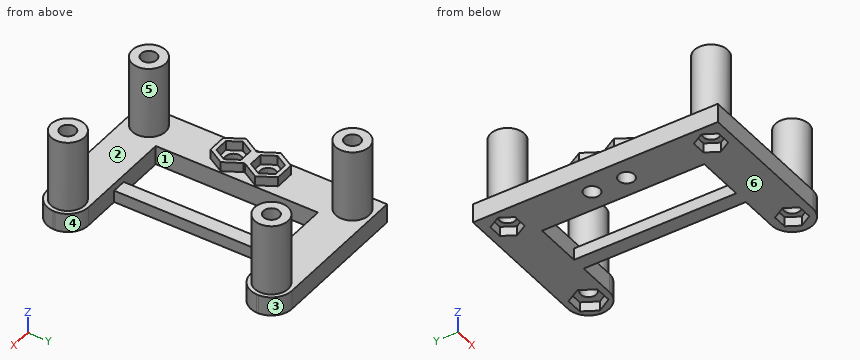
Autodesk Inventor part; units mm, degrees
ref_plane "YZ Plane" through (0, 0, 0) normal (1, 0, 0) x (0, 1, 0)
ref_plane "XZ Plane" through (0, 0, 0) normal (0, 1, 0) x (-1, 0, 0)
ref_plane "XY Plane" through (0, 0, 0) normal (0, 0, 1) x (1, 0, 0)
sketch "Sketch1" plane through (0, 0, 0) normal (0, 0, 1) x (1, 0, 0)
  line L0 (0, 0) -> (41.5, 0)
  line L1 (41.5, 0) -> (41.5, -73)
  line L2 (41.5, -73) -> (0, -73)
  line L3 (0, -73) -> (0, 0)
  line L4 (0, -73) -> (3.11, -73)
  line L5 (0, -73) -> (3.11, -73) construction
  line L6 (3.11, -73) -> (3.11, -69.85)
  line L7 (3.11, -73) -> (6.26, -73) construction
  line L8 (3.11, -69.85) -> (14.54, -69.85)
  line L9 (14.54, -69.85) -> (19.65, -69.85)
  line L10 (19.65, -69.85) -> (31.08, -69.85)
  circle A0 centre (3.11, -69.85) radius 1.6
  circle A1 centre (14.54, -69.85) radius 1.6
  circle A2 centre (19.65, -69.85) radius 1.6
  circle A3 centre (31.08, -69.85) radius 1.6
  line L11 (3.11, -69.85) -> (3.11, -55.42)
  line L12 (3.11, -69.85) -> (17.54, -69.85) construction
  line L13 (0, -73) -> (4.33, -73)
  line L14 (0, -73) -> (4.33, -73) construction
  line L15 (4.33, -73) -> (4.33, -53.49)
  line L16 (3.11, -55.42) -> (6.6479, -55.42)
  circle A4 centre (4.33, -55.42) radius 1.651
  line L17 (4.33, -55.42) -> (4.33, -37.69)
  line L18 (4.33, -55.42) -> (22.06, -55.42) construction
  line L19 (4.33, -55.42) -> (29.68, -55.42)
  line L20 (4.33, -55.42) -> (29.68, -55.42) construction
  circle A5 centre (4.33, -37.69) radius 1.651
  circle A6 centre (29.68, -55.42) radius 1.651
  line L21 (4.33, -37.69) -> (39.0376, -37.69)
  line L22 (29.68, -55.42) -> (29.68, -25.3245)
  circle A7 centre (29.68, -37.69) radius 1.651
  line L23 (4.33, -37.69) -> (4.33, -30.44)
  line L24 (4.33, -37.69) -> (11.58, -37.69) construction
  line L25 (4.33, -30.44) -> (4.33, -12.71)
  line L26 (4.33, -30.44) -> (29.68, -30.44)
  line L27 (4.33, -30.44) -> (29.68, -30.44) construction
  line L28 (4.33, -12.71) -> (29.68, -12.71)
  circle A8 centre (29.68, -12.71) radius 1.651
  circle A9 centre (4.33, -12.71) radius 1.651
  circle A10 centre (4.33, -30.44) radius 1.651
  circle A11 centre (29.68, -30.44) radius 1.651
  line L29 (29.68, -12.71) -> (29.68, -11.3536)
  dimension "d0" = 41.5
  dimension "d1" = 73
  dimension "d2" = 3.11
  dimension "d3" = 0
  dimension "d4" = 3.15
  dimension "d5" = 90
  dimension "d6" = 11.43
  dimension "d7" = 90
  dimension "d9" = 5.11
  dimension "d10" = 11.43
  dimension "d11" = 180
  dimension "d12" = 3.2
  dimension "d13" = 3.2
  dimension "d14" = 3.2
  dimension "d15" = 3.2
  dimension "d18" = 14.43
  dimension "d19" = 90
  dimension "d20" = 4.33
  dimension "d21" = 0
  dimension "d22" = 3.302
  dimension "d23" = 17.73
  dimension "d24" = 90
  dimension "d25" = 25.35
  dimension "d26" = 0
  dimension "d27" = 3.302
  dimension "d28" = 3.302
  dimension "d29" = 3.302
  dimension "d30" = 7.25
  dimension "d31" = 90
  dimension "d32" = 17.73
  dimension "d33" = 180
  dimension "d34" = 25.35
  dimension "d35" = 0
  dimension "d36" = 25.35
  dimension "d37" = 3.302
  dimension "d38" = 3.302
  dimension "d39" = 3.302
  dimension "d40" = 3.302
extrude "Extrusion2" add sketch "Sketch1" along normal blind 4 contours L0 L1 L2 L15 A0 A4 L16 L19 A6 L22 A7 A11 L26 A10 L23 A5 L17 L11 L6 L3 | L6 A0 L15 L2 | L11 A4 L15 A0 | L15 L17 A5 L21 A7 L22 A6 L19 L16 A4 | L23 A10 L26 A11 L22 A7 L21 A5
sketch "Sketch3" plane through (0, 0, 4) normal (0, 0, 1) x (1, 0, 0)
  circle A0 centre (4.33, -55.42) radius 1.651
  circle A1 centre (4.33, -55.42) radius 3.5
  circle A2 centre (29.68, -55.42) radius 1.651
  circle A3 centre (29.68, -55.42) radius 3.5
  circle A4 centre (4.33, -12.71) radius 1.651
  circle A5 centre (4.33, -12.71) radius 3.5
  circle A6 centre (29.68, -12.71) radius 1.651
  circle A7 centre (29.68, -12.71) radius 3.5
  point P0 (0, 0)
  dimension "d46" = 7
  dimension "d47" = 7
  dimension "d48" = 7
  dimension "d49" = 7
extrude "Extrusion4" add sketch "Sketch3" along normal blind 15
sketch "Sketch8" plane through (0, 0, 0) normal (0, 0, -1) x (-1, 0, 0)
  circle A0 centre (-4.33, -12.71) radius 1.651
  circle A1 centre (-4.33, -12.71) radius 3
  circle A2 centre (-29.68, -12.71) radius 1.651
  circle A3 centre (-29.68, -12.71) radius 3
  circle A4 centre (-29.68, -55.42) radius 1.651
  circle A5 centre (-29.68, -55.42) radius 3
  circle A6 centre (-4.33, -55.42) radius 1.651
  circle A7 centre (-4.33, -55.42) radius 3
  line L0 (-1.33, -12.71) -> (-2.83, -15.3081)
  line L1 (-2.83, -15.3081) -> (-5.83, -15.3081)
  line L2 (-5.83, -15.3081) -> (-7.33, -12.71)
  line L3 (-7.33, -12.71) -> (-5.83, -10.1119)
  line L4 (-5.83, -10.1119) -> (-2.83, -10.1119)
  line L5 (-2.83, -10.1119) -> (-1.33, -12.71)
  circle A8 centre (-29.68, -12.71) radius 3.5
  line L6 (-26.18, -12.6978) -> (-27.9194, -15.735)
  line L7 (-27.9194, -15.735) -> (-31.4194, -15.7472)
  line L8 (-31.4194, -15.7472) -> (-33.18, -12.7222)
  line L9 (-33.18, -12.7222) -> (-31.4406, -9.685)
  line L10 (-31.4406, -9.685) -> (-27.9406, -9.6728)
  line L11 (-27.9406, -9.6728) -> (-26.18, -12.6978)
  line L12 (-26.68, -55.42) -> (-28.18, -58.0181)
  line L13 (-28.18, -58.0181) -> (-31.18, -58.0181)
  line L14 (-31.18, -58.0181) -> (-32.68, -55.42)
  line L15 (-32.68, -55.42) -> (-31.18, -52.8219)
  line L16 (-31.18, -52.8219) -> (-28.18, -52.8219)
  line L17 (-28.18, -52.8219) -> (-26.68, -55.42)
  line L18 (-1.3301, -55.3946) -> (-2.808, -58.0053)
  line L19 (-2.808, -58.0053) -> (-5.8079, -58.0307)
  line L20 (-5.8079, -58.0307) -> (-7.3299, -55.4454)
  line L21 (-7.3299, -55.4454) -> (-5.852, -52.8347)
  line L22 (-5.852, -52.8347) -> (-2.8521, -52.8093)
  line L23 (-2.8521, -52.8093) -> (-1.3301, -55.3946)
  point P0 (0, 0)
  dimension "d53" = 6
  dimension "d55" = 6
  dimension "d56" = 6
  dimension "d54" = 6
extrude "Extrusion5" cut sketch "Sketch8" against normal blind 2 contours L0 L1 L2 L3 L4 L5 | A2 | A3 | L12 L13 L14 L15 L16 L17 | L18 L19 L20 L21 L22 L23 | L6 L7 L8 L9 L10 L11
sketch "Sketch9" plane through (0, 0, 4) normal (0, 0, 1) x (1, 0, 0)
  circle A0 centre (4.33, -30.44) radius 1.651
  circle A1 centre (4.33, -30.44) radius 1.651
  circle A2 centre (4.33, -37.69) radius 1.651
  circle A3 centre (4.33, -37.69) radius 1.651
  line L0 (7.33, -30.44) -> (5.83, -33.0381)
  line L1 (5.83, -33.0381) -> (2.83, -33.0381)
  line L2 (2.83, -33.0381) -> (1.33, -30.44)
  line L3 (1.33, -30.44) -> (2.83, -27.8419)
  line L4 (2.83, -27.8419) -> (5.83, -27.8419)
  line L5 (5.83, -27.8419) -> (7.33, -30.44)
  line L6 (7.33, -37.69) -> (5.83, -40.2881)
  line L7 (5.83, -40.2881) -> (2.83, -40.2881)
  line L8 (2.83, -40.2881) -> (1.33, -37.69)
  line L9 (1.33, -37.69) -> (2.83, -35.0919)
  line L10 (2.83, -35.0919) -> (5.83, -35.0919)
  line L11 (5.83, -35.0919) -> (7.33, -37.69)
  line L12 (8.33, -30.44) -> (6.33, -33.9041)
  line L13 (6.33, -33.9041) -> (2.33, -33.9041)
  line L14 (2.33, -33.9041) -> (0.33, -30.44)
  line L15 (0.33, -30.44) -> (2.33, -26.9759)
  line L16 (2.33, -26.9759) -> (6.33, -26.9759)
  line L17 (6.33, -26.9759) -> (8.33, -30.44)
  line L18 (8.33, -37.69) -> (6.33, -41.1541)
  line L19 (6.33, -41.1541) -> (2.33, -41.1541)
  line L20 (2.33, -41.1541) -> (0.33, -37.69)
  line L21 (0.33, -37.69) -> (2.33, -34.2259)
  line L22 (2.33, -34.2259) -> (6.33, -34.2259)
  line L23 (6.33, -34.2259) -> (8.33, -37.69)
  line L24 (6.33, -33.9041) -> (6.33, -34.2259)
  line L25 (2.33, -33.9041) -> (2.33, -34.2259)
  point P0 (0, 0)
  dimension "d59" = 3.302
  dimension "d60" = 3.302
extrude "Extrusion6" add sketch "Sketch9" along normal blind 2 contours L12 L13 L14 L15 L16 L17 | L24 L22 L25 L13 | L23 L18 L19 L20 L21 L22
sketch "Sketch10" plane through (0, 0, 0) normal (0, 0, -1) x (-1, 0, 0)
  circle A0 centre (-4.33, -55.42) radius 1.651
  circle A1 centre (-4.33, -12.71) radius 3.5
  circle A2 centre (-4.33, -12.71) radius 4.33
  line L0 (-4.33, -8.38) -> (6.0992, -8.38)
  line L1 (-4.33, -8.38) -> (-46.273, -8.38)
  circle A3 centre (-29.68, -55.42) radius 1.651
  circle A4 centre (-29.68, -12.71) radius 1.651
  circle A5 centre (-29.68, -12.71) radius 4.33
  line L2 (-34.01, -12.71) -> (-34.01, 23.2585)
  circle A6 centre (-4.33, -55.42) radius 4.33
  line L3 (-34.01, -12.71) -> (-34.01, -66.3278)
  line L4 (-4.33, -59.75) -> (-38.3543, -59.75)
  circle A7 centre (-29.68, -55.42) radius 4.33
  line L5 (-29.68, -55.42) -> (-29.68, -12.71)
  circle A8 centre (-4.33, -12.71) radius 1.651
  line L6 (-4.33, -12.71) -> (-29.68, -12.71)
  line L7 (-18.2288, -59.75) -> (-46.273, -59.75)
  line L8 (-46.273, -59.75) -> (-46.273, -78.0952)
  line L9 (-46.273, -78.0952) -> (-18.2288, -78.0952)
  line L10 (-18.2288, -78.0952) -> (-18.2288, -59.75)
  line L11 (-18.2288, -59.75) -> (2.2846, -59.75)
  line L12 (2.2846, -59.75) -> (2.2846, -79.2844)
  line L13 (2.2846, -79.2844) -> (-18.2288, -79.2844)
  line L14 (-18.2288, -79.2844) -> (-18.2288, -59.75)
  line L15 (-34.01, -59.75) -> (-49.3705, -59.75)
  line L16 (-49.3705, -59.75) -> (-49.3705, 18.5259)
  line L17 (-49.3705, 18.5259) -> (-34.01, 18.5259)
  line L18 (-34.01, 18.5259) -> (-34.01, -59.75)
  line L19 (-34.01, -8.38) -> (8.0076, -8.38)
  line L20 (8.0076, -8.38) -> (8.0076, 15.8503)
  line L21 (8.0076, 15.8503) -> (-34.01, 15.8503)
  line L22 (-34.01, 15.8503) -> (-34.01, -8.38)
  point P0 (0, 0)
extrude "Extrusion7" cut sketch "Sketch10" along normal mid plane 100 contours L1 L2 L21 L20 L19 L0 | L2 L3 L4 L7 L15 L16 L17 | L4 L10 L9 L8 L7 | L4 L11 L12 L13 L14 L10
sketch "Sketch11" plane through (0, 0, 0) normal (0, 0, -1) x (-1, 0, 0)
  line L0 (-34.01, -59.75) -> (0, -59.75)
  line L1 (0, -8.38) -> (-34.01, -8.38)
  circle A0 centre (-4.33, -55.42) radius 1.651
  circle A1 centre (-4.33, -55.42) radius 4.3403
  circle A2 centre (-4.33, -12.71) radius 1.651
  circle A3 centre (-4.33, -12.71) radius 4.3403
  line L2 (-4.3352, -51.0797) -> (-29.68, -51.0797)
  line L3 (-29.68, -59.75) -> (-4.3352, -59.75)
  line L4 (-4.3352, -59.75) -> (-4.3352, -51.0797)
  line L5 (-4.3352, -17.0503) -> (-29.68, -17.0503)
  line L6 (-29.68, -8.38) -> (-4.3352, -8.38)
  line L7 (-4.3352, -8.38) -> (-4.3352, -17.0503)
  line L8 (-4.3352, -51.0797) -> (-8.6703, -51.0797)
  line L9 (-8.6703, -51.0797) -> (-8.6703, -12.7152)
  line L10 (-8.6703, -12.7152) -> (-4.3352, -12.7152)
  line L11 (-4.3352, -12.7152) -> (-4.3352, -51.0797)
  line L12 (-34.01, -8.38) -> (-34.01, -59.75)
  line L13 (-8.6703, -17.0503) -> (-34.01, -17.0503)
  line L14 (-34.01, -17.0503) -> (-34.01, -51.0797)
  line L15 (-34.01, -51.0797) -> (-8.6703, -51.0797)
  line L16 (-8.6703, -51.0797) -> (-8.6703, -17.0503)
  line L17 (-29.68, -59.75) -> (-36.7019, -59.75)
  line L18 (-36.7019, -59.75) -> (-36.7019, -51.0797)
  line L19 (-36.7019, -51.0797) -> (-29.68, -51.0797)
  line L20 (-29.68, -17.0503) -> (-34.01, -17.0503)
  line L21 (-34.01, -17.0503) -> (-34.01, -8.38)
  line L22 (-34.01, -8.38) -> (-29.68, -8.38)
  arc A4 (-29.68, -51.0797) -> (-29.68, -59.75) centre (-29.68, -55.4148) ccw
  arc A5 (-29.68, -8.38) -> (-29.68, -17.0503) centre (-29.68, -12.7152) ccw
  line L23 (-29.68, -17.0503) -> (-40.5173, -17.0503)
  line L24 (-40.5173, -17.0503) -> (-40.5173, -8.38)
  line L25 (-40.5173, -8.38) -> (-29.68, -8.38)
  line L26 (-8.6703, -51.0797) -> (-41.5169, -51.0797)
  line L27 (-41.5169, -51.0797) -> (-41.5169, -17.0503)
  line L28 (-41.5169, -17.0503) -> (-8.6703, -17.0503)
  line L29 (-8.6703, -17.0503) -> (-8.6703, -51.0797)
  arc A6 (-29.68, -8.38) -> (-29.68, -17.0503) centre (-29.68, -12.7152) ccw
  line L30 (-29.68, -8.38) -> (-34.01, -8.38)
  point P0 (0, 0)
  point P1 (-29.68, -55.42)
extrude "Extrusion8" cut sketch "Sketch11" along normal mid plane 100 contours L12 A4 L0 | L17 L18 L19 L12 A4 | L12 L15 A4 | L12 L13 L5 L9 L2 L15 | L23 L24 L25 L12 A5 | L12 A5 L13 | L12 L1 A5
sketch "Sketch12" plane through (0, 0, 0) normal (0, 0, -1) x (-1, 0, 0)
  line L0 (-29.68, -51.0797) -> (-8.6703, -51.0797)
  line L1 (-8.6703, -17.0503) -> (-29.68, -17.0503)
  line L2 (-8.6703, -51.0797) -> (-18.6703, -51.0797)
  line L3 (-18.6703, -51.0797) -> (-18.6703, -17.0503)
  line L4 (-18.6703, -17.0503) -> (-8.6703, -17.0503)
  line L5 (-8.6703, -17.0503) -> (-8.6703, -51.0797)
  line L6 (-18.6703, -17.0503) -> (-21.6703, -17.0503)
  line L7 (-21.6703, -17.0503) -> (-21.6703, -51.0797)
  line L8 (-21.6703, -51.0797) -> (-18.6703, -51.0797)
  line L9 (-18.6703, -51.0797) -> (-18.6703, -17.0503)
  point P0 (0, 0)
  dimension "d71" = 10
  dimension "d72" = 3
extrude "Extrusion9" add sketch "Sketch12" against normal blind 2.5 contours L7 L1 L3 L0
properties part number "mountMount"
CAD build for the part. Positions are in the model's coordinates, mm. Face numbers are marked on the shaded views. A direction names the side the tool comes from. Round coordinates to 2 decimals unless told otherwise and drop trailing zeros. Write each loop counter-clockwise with the first axis right and the second up, starting at its lowest first coordinate (ties: lowest second). Pieces come first, ordered by that corner, then holes. Notation, with made-up numbers: (34, 35.25) - (43, 35.25) arc R21 cw to (43, 63.25) - close; hole circle Ø10 at (71, -4). An arc over 180 degrees is marked (long way). Return JSON: item names as keys, results as strings. Group by question number.
Item 1: 3-axis set-ups, long thin cutter, end or side, ignore diameter. For the marked faces 1, 2 and 3: which of +Z, -Z, +X, -X, +Y, -Y reach the whole face in a straight line?
Item 2: Flat gauge pins, fed straight in: pin 1 Ø0.6 at (x, z) = (4, 5) entering from +Y; pin 2 Ø3 at (x, y) = (31, -12) entering from -Z; pin 3 Ø9 at (x, y) = (4.5, -33) entering from +Z. Where does each tip first touch, or does it go through?
Item 3: Band-saw the part on A-A on z = 13. List the corners of the cut face in (x, y), plus the area to 3 significant figures.
Item 4: Band-saw the part on C-C on y = -25. List the corners of the cut face in (x, z), plus the area to 3 significant figures.
Item 5: Band-saw the part on B-B on x = 10.5. List the corners of the cut face in (y, z), plus the area to 3 significant figures.
Item 6: Band-saw the part on D-D on x = 4.33. State how many separate pieces and enclosed holes the cut face has, plus the area to 3 significant figures.
Item 7: Probe probe 1 along Y at (x, z) = (4.33, 1.5); probe 2 along Y at (x, z) = (4.33, 3); probe 3 along Y at (x, z) = (29.68, 14). List the from-to ranges inside material, lowest first.
Item 8: Mould opens along X. For the marked faces 4, 5 and 6 say: +X half, -X half, draft (parallel to the pull), parting line (faces both ways), or undercut.
Resolved:
{
 "1": {"face 1": "+Z, -Z", "face 2": "+Z", "face 3": "+Z, -Z, +X, +Y"},
 "2": {"pin 1": "stops at y = -9.21", "pin 2": "stops at z = 2", "pin 3": "stops at z = 6"},
 "3": {"outline": "circle Ø7 at (4.33, -55.42); circle Ø7 at (4.33, -12.71); circle Ø7 at (29.68, -55.42); circle Ø7 at (29.68, -12.71); hole circle Ø3.3 at (4.33, -55.42); hole circle Ø3.3 at (4.33, -12.71); hole circle Ø3.3 at (29.68, -55.42); hole circle Ø3.3 at (29.68, -12.71)", "area": "120 mm²"},
 "4": {"outline": "(0, 0) - (8.67, 0) - (8.67, 4) - (0, 4) - close; (18.67, 0) - (21.67, 0) - (21.67, 2.5) - (18.67, 2.5) - close", "area": "42.2 mm²"},
 "5": {"outline": "(-59.75, 0) - (-51.08, 0) - (-51.08, 4) - (-59.75, 4) - close; (-17.05, 0) - (-8.38, 0) - (-8.38, 4) - (-17.05, 4) - close", "area": "69.4 mm²"},
 "6": {"separate pieces": "5", "enclosed holes": "0", "area": "264 mm²"},
 "7": {"probe 1": "y = -59.75 to -58.02, -52.82 to -39.34, -36.04 to -32.09, -28.79 to -15.31, -10.11 to -8.38", "probe 2": "y = -59.75 to -57.07, -53.77 to -39.34, -36.04 to -32.09, -28.79 to -14.36, -11.06 to -8.38", "probe 3": "y = -58.92 to -57.07, -53.77 to -51.92, -16.21 to -14.36, -11.06 to -9.21"},
 "8": {"face 4": "+X half", "face 5": "undercut", "face 6": "draft"}
}
